CAD build for the part. Positions are in the model's coordinates, mm. Face numbers are marked on the shaded views. A direction names the side the tool comes from. Round coordinates to 2 decimals unless told otherwise and drop trailing zeros. Order: outer loops, then holes, each group sorted by start corner. A loop starts at its lowest first (then second) coordinate and runs counter-clockwise, first axis right, second up. Notation, with made-up numbers: (73, 6) - (88, 6) arc R21 cw to (88, 13) - close; hole circle Ø11 at (-10, -19). An arc over 180 degrees is marked (long way). Write item = value, one per line.
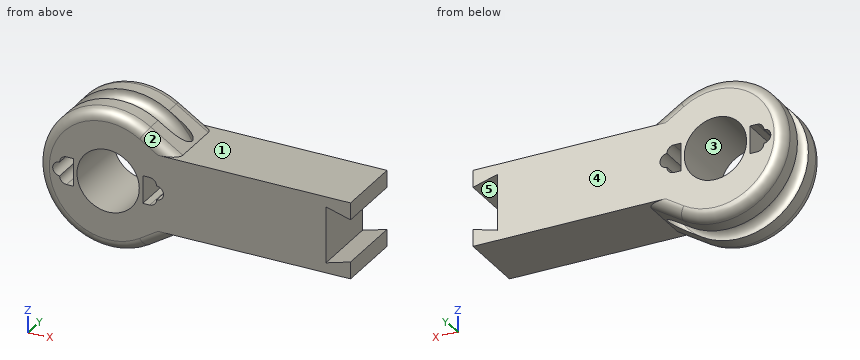
from build123d import *

# Parameters (mm, degrees)
SKETCH1_R           = 4.5
BOSS_EXTRUDE2_DEPTH = 10
FILLET2_R           = 1.5


with BuildPart() as part:
    # Sketch1 → Boss-Extrude2 (new body)
    with BuildSketch(Plane(origin=(0, 0, 0), x_dir=(1, 0, 0), z_dir=(0, 1, 0))):
        with BuildLine():
            Line((35, 5.500000000000003), (10, 5.500000000000003))
            Line((10, 5.500000000000003), (5.355086372360837, 8.445297504798466))
            ThreePointArc((5.355086372360837, 8.445297504798466), (-10, 1.11e-14), (5.355086372360817, -8.445297504798482))
            Line((5.355086372360817, -8.445297504798482), (10, -5.499999999999997))
            Line((10, -5.499999999999997), (34.99999999999999, -5.499999999999997))
            Line((34.99999999999999, -5.499999999999997), (35, -3.05))
            Line((35, -3.05), (31.449999999999992, -4.050000000000006))
            Line((31.449999999999992, -4.050000000000006), (31.450000000000006, 4.049999999999974))
            Line((31.450000000000006, 4.049999999999973), (35, 3.05))
            Line((35, 3.05), (35, 5.500000000000003))
        make_face()
        with BuildLine():
            Line((-5, 2), (-4.999999999999999, -2))
            Line((-4.999999999999999, -2), (-5.999999999999992, -2))
            ThreePointArc((-5.999999999999992, -1.9999999999999998), (-6.707106781186546, -1.7071067811865475), (-6.999999999999999, -0.9999999999999932))
            ThreePointArc((-6.999999999999999, -1.0000000000000002), (-7.999999999999999, -7.6e-16), (-7, 0.9999999999999993))
            ThreePointArc((-7, 0.9999999999999923), (-6.707106781186547, 1.707106781186547), (-5.999999999999993, 2))
            Line((-5.999999999999993, 1.9999999999999996), (-5, 2))
        make_face(mode=Mode.SUBTRACT)
        with Locations(Location((0, 0, 0), (0, 0, 270))):
            Circle(SKETCH1_R, mode=Mode.SUBTRACT)
        with BuildLine():
            Line((4.999999999999999, -2), (5, 2))
            Line((5, 2), (5.999999999999993, 1.9999999999999996))
            ThreePointArc((5.999999999999993, 1.9999999999999998), (6.707106781186548, 1.707106781186547), (7, 0.9999999999999923))
            ThreePointArc((7, 0.9999999999999993), (7.707106781186547, 0.7071067811865467), (7.999999999999999, -4.3e-16))
            ThreePointArc((7.999999999999999, -6.8e-16), (7.707106781186546, -0.707106781186548), (6.999999999999999, -1.0000000000000002))
            ThreePointArc((6.999999999999999, -0.9999999999999932), (6.707106781186546, -1.7071067811865475), (5.999999999999992, -1.9999999999999998))
            Line((5.999999999999992, -2), (4.999999999999999, -2))
        make_face(mode=Mode.SUBTRACT)
    extrude(amount=BOSS_EXTRUDE2_DEPTH)

    # Sketch4 → Cut-Revolve3 (revolve, cut)
    with BuildSketch(Plane(origin=(-6.666818896321271, 16.53530046448365, 0), x_dir=(0, 1, 0), z_dir=(0, 0, 1)), mode=Mode.PRIVATE) as cut_revolve3_sk:
        with BuildLine():
            ThreePointArc((-13.035300464483651, 3.333181103678728), (-11.535300464483651, 1.833181103678728), (-10.035300464483651, 3.333181103678728))
            add(Edge.make_bspline(
                [(-10.035300464483651, 3.333181103678728), (-10.035300464483651, 4.483181103678728), (-11.535300464483651, 4.483181103678728), (-13.035300464483651, 4.483181103678727), (-13.035300464483651, 3.333181103678728)],
                knots=[0, 0, 0, 1.5707963267948966, 1.5707963267948966, 3.141592653589793, 3.141592653589793, 3.141592653589793], degree=2, weights=[1, 0.7071067811865476, 1, 0.7071067811865476, 1]))
        make_face()
    revolve(cut_revolve3_sk.sketch.rotate(Axis((0, 0, 0), (0, 1, 0)), 237.621587486), axis=Axis((0, 0, 0), (0, 1, 0)), mode=Mode.SUBTRACT)

    # Fillet2
    fillet2_edges = [part.edges().sort_by_distance(p)[0] for p in [
        (7.677543186180419, 0, -6.972648752399234),
        (-10, 0, -1.11e-14),
        (7.677543186180419, 10, -6.972648752399234),
        (-10, 10, -1.11e-14),
        (7.677543186180408, 0, 6.972648752399239),
        (7.677543186180408, 10, 6.972648752399239),
    ]]
    fillet(fillet2_edges, radius=FILLET2_R)


solid = part.part
(1) Band-saw the part on A-A on x = 0. List the corners of the cut face in (y, z).
Solved:
outline = (0, -8.5) arc R1.5 ccw to (1.5, -10) - (3.5, -10) arc R1.5 cw to (6.5, -10) - (8.5, -10) arc R1.5 ccw to (10, -8.5) - (10, -4.5) - (0, -4.5) - close; (0, 4.5) - (10, 4.5) - (10, 8.5) arc R1.5 ccw to (8.5, 10) - (6.5, 10) arc R1.5 cw to (3.5, 10) - (1.5, 10) arc R1.5 ccw to (0, 8.5) - close
(2) Probe line 1 along X through (y, z) = (3, 0); line 2 along X through (y, z) = (5.5, 0); line 3 along X through (y, z) = (4.25, 0). List the from-to ranges inside material, lowest first.
Solved:
line_1 = -10 to -8, -5 to -4.5, 4.5 to 5, 8 to 31.45
line_2 = -8.59 to -8, -5 to -4.5, 4.5 to 5, 8 to 8.59, 11.08 to 31.45
line_3 = -8.7 to -8, -5 to -4.5, 4.5 to 5, 8 to 8.7, 11 to 31.45
(3) Tool access for the marked faces 4 and 5: list every direction of +Z, -Z, +X, -X, +Y, -Y with a clear straight run to the whole face (end or side of a thin tool).
Solved:
face_4 = +Z, -Z, +X, -X, +Y
face_5 = +Y, -Y
(4) Pull direction X, two halves, no side cores. Call the marked faces 1, 2 and 3: released by +X, released by -X, zero draft, split by the parting line, or undercut.
Solved:
face_1 = zero draft
face_2 = released by +X
face_3 = undercut
(5) Band-saw the part on B-B on y = 2. List the corners of the cut face in (x, z), plus the area to 3 significant figures.
Solved:
outline = (5.36, -8.45) - (10, -5.5) - (35, -5.5) - (35, -3.05) - (31.45, -4.05) - (31.45, 4.05) - (35, 3.05) - (35, 5.5) - (10, 5.5) - (5.36, 8.45) arc R10 ccw (long way) to start; hole (-7, -1) arc R1 ccw to (-6, -2) - (-5, -2) - (-5, 2) - (-6, 2) arc R1 ccw to (-7, 1) arc R1 ccw to start; hole circle Ø9 at (0, 0); hole (5, -2) - (6, -2) arc R1 ccw to (7, -1) arc R1 ccw to (7, 1) arc R1 ccw to (6, 2) - (5, 2) - close
area = 491 mm²
(6) Drop flat-ended pins along their axis: pin 1 (6 mm diameter, centred on x = 29.5, y = 4.5, fed in from +Z); pin 2 (1.1 mm diameter, centred on x = -5.5, y = 6.5, fed in from -Z); pin 3 (3 mm diameter, centred on y = 7.5, z = 7, fed in from -X). Give the stop position or say it passes through.
Solved:
pin_1 = 5.5
pin_2 = -8.69
pin_3 = -8.35
(7) Band-saw the part on C-C on x = 28. List the corners of the cut face in (y, z), plus the area to 3 significant figures.
Solved:
outline = (0, -5.5) - (10, -5.5) - (10, 5.5) - (0, 5.5) - close
area = 110 mm²
